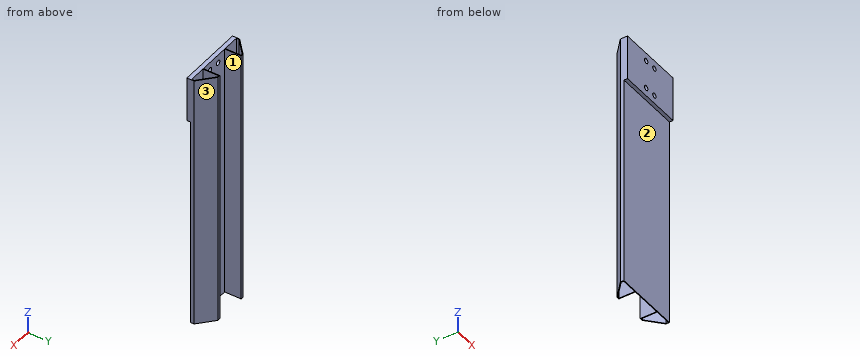
```python
from build123d import *

# Parameters (mm, degrees)
CROQUIS2_W              = 94
CROQUIS2_H              = 24
SALIENTE_EXTRUIR1_DEPTH = 360
CROQUIS4_W              = 44
CROQUIS4_H              = 23
CORTAR_EXTRUIR2_DEPTH   = 360
CORTAR_EXTRUIR3_DEPTH   = 360
CORTAR_EXTRUIR5_DEPTH   = 360
CROQUIS8_W              = 94
CROQUIS8_H              = 63
SALIENTE_EXTRUIR2_DEPTH = 5
CROQUIS9_R              = 3.5
CORTAR_EXTRUIR6_DEPTH   = 30


with BuildPart() as part:
    # Croquis2 → Saliente-Extruir1 (new body)
    with BuildSketch(Plane.XY):
        with Locations((47, -12)):
            Rectangle(CROQUIS2_W, CROQUIS2_H)
    extrude(amount=SALIENTE_EXTRUIR1_DEPTH)

    # Croquis4 → Cortar-Extruir2 (cut)
    with BuildSketch(Plane(origin=(0, 0, 0), x_dir=(-1, 0, 0), z_dir=(0, 0, -1))):
        Polygon((-94, 0), (-94, -19), (-73, 0), align=None)
        with Locations((-47, -11.5)):
            Rectangle(CROQUIS4_W, CROQUIS4_H)
        Polygon((0, 0), (-21, 0), (0, -19), align=None)
    extrude(amount=-CORTAR_EXTRUIR2_DEPTH, mode=Mode.SUBTRACT)

    # Croquis6 → Cortar-Extruir3 (cut)
    with BuildSketch(Plane(origin=(0, 0, 0), x_dir=(-1, 0, 0), z_dir=(0, 0, -1))):
        Polygon((-70, -23), (-70, -1), (-72.614757657, -1), (-93, -19.443790691), (-93, -23), align=None)
    extrude(amount=-CORTAR_EXTRUIR3_DEPTH, mode=Mode.SUBTRACT)

    # Croquis7 → Cortar-Extruir5 (cut)
    with BuildSketch(Plane(origin=(0, 0, 0), x_dir=(-1, 0, 0), z_dir=(0, 0, -1))):
        Polygon((-1, -19.443790691), (-21.385242343, -1), (-24, -1), (-24, -23), (-1, -23), align=None)
    extrude(amount=-CORTAR_EXTRUIR5_DEPTH, mode=Mode.SUBTRACT)

    # Croquis8 → Saliente-Extruir2 (add)
    with BuildSketch(Plane.XZ.offset(24)):
        with Locations((47, 328.5)):
            Rectangle(CROQUIS8_W, CROQUIS8_H)
    extrude(amount=SALIENTE_EXTRUIR2_DEPTH)

    # Croquis9 → Cortar-Extruir6 (cut, through all)
    with BuildSketch(Plane.XZ.offset(29)):
        with Locations((38.5, 348.5)):
            Circle(CROQUIS9_R)
        with Locations((55.5, 348.5)):
            Circle(CROQUIS9_R)
        with Locations((38.5, 308.5)):
            Circle(CROQUIS9_R)
        with Locations((55.5, 308.5)):
            Circle(CROQUIS9_R)
    extrude(amount=-CORTAR_EXTRUIR6_DEPTH, mode=Mode.SUBTRACT)


solid = part.part
```
Source: CAD feature listing. Evaluate the final solid. Frame: model axes, mm. Face numbers are marked on the shaded views. Round coordinates to 2 decimals unless told otherwise and drop trailing zeros. Loops run counter-clockwise (first coordinate to the right, second up) from the corner with the lowest first, then second, coordinate; pieces in that order, holes last.
1. Section query B-B on x = 38.5. Output: boundary loops of the cut face in (y, z).
2. Section query A-A on z = 308.5. Output: boundary loops of the cut face in (x, y).
3. Ray query, L1, parallel to Z at x = 55.5, y = -26.7; L2, parallel to X at y = -26.1, z = 308.5; L3, parallel to X at y = -14.75, z = 58. Return the intervals inside material, ascending.
4. Mould query, pull axis X, two halves, no side actions, for the marked faces 1, 2 and 3. Classes: released by +X, released by -X, zero draft, split by the parting line, or undercut.
5. Section query D-D on y = -6.25. Output: boundary loops of the cut face in (x, z).
6. Contact query for flat-ended pins moving along their axis: pin 1 (13 mm diameter, centred on x = 44, z = 107, fed in from +Y); pin 2 (5 mm diameter, centred on x = 75, z = 293.5, fed in from -Y); pin 3 (5.5 mm diameter, centred on x = 38.5, z = 348.5, fed in from +Y); pin 4 (1.8 mm diameter, centred on y = -21, z = 156, fed in from -X). Output: stop coordinate, or through.
7. Section query C-C on z = 222.5. Output: boundary loops of the cut face in (x, y), and give its area (3 significant figures).
Answers below:
1. outline: (-29, 297) - (-24, 297) - (-24, 0) - (-23, 0) - (-23, 305) - (-29, 305) - close; (-29, 312) - (-23, 312) - (-23, 345) - (-29, 345) - close; (-29, 352) - (-23, 352) - (-23, 360) - (-29, 360) - close
2. outline: (0, -29) - (35, -29) - (35, -23) - (25, -23) - (25, 0) - (21, 0) - (0, -19) - close; (42, -29) - (52, -29) - (52, -23) - (42, -23) - close; (59, -29) - (94, -29) - (94, -19) - (73, 0) - (69, 0) - (69, -23) - (59, -23) - close; hole (1, -23) - (24, -23) - (24, -1) - (21.39, -1) - (1, -19.44) - close; hole (70, -23) - (93, -23) - (93, -19.44) - (72.61, -1) - (70, -1) - close
3. L1: z = 297 to 305, 312 to 345, 352 to 360
3. L2: x = 0 to 35, 42 to 52, 59 to 94
3. L3: x = 4.7 to 6.19, 24 to 25, 69 to 70, 87.81 to 89.3
4. face 1: undercut
4. face 2: zero draft
4. face 3: released by +X
5. outline: (14.09, 0) - (15.58, 0) - (15.58, 360) - (14.09, 360) - close; (24, 0) - (25, 0) - (25, 360) - (24, 360) - close; (69, 0) - (70, 0) - (70, 360) - (69, 360) - close; (78.42, 0) - (79.91, 0) - (79.91, 360) - (78.42, 360) - close
6. pin 1: stops at y = -23
6. pin 2: stops at y = -24
6. pin 3: passes through
6. pin 4: stops at x = 0
7. outline: (0, -24) - (94, -24) - (94, -19) - (73, 0) - (69, 0) - (69, -23) - (25, -23) - (25, 0) - (21, 0) - (0, -19) - close; hole (1, -23) - (24, -23) - (24, -1) - (21.39, -1) - (1, -19.44) - close; hole (70, -23) - (93, -23) - (93, -19.44) - (72.61, -1) - (70, -1) - close
7. area: 209 mm2
